Geometry: final body of the model. Coordinates: model frame, mm. A direction names the side the tool comes from. Coordinates: 2 decimals unless noted, no trailing zeros. Write each loop counter-clockwise with the first axis right and the second up, starting at its lowest first coordinate (ties: lowest second). Pieces come first, ordered by that corner, then holes.
from build123d import *

# Parameters (mm, degrees)
SKETCH_1_W          = 31
SKETCH_1_H          = 12.6
EXTRUDE_1_DEPTH     = 1
SKETCH_2_R          = 2.5
EXTRUDE_2_DEPTH     = 6
SKETCH_3_R          = 1.5
EXTRUDE_3_DEPTH     = 5.5
DOME_1_FACE_RADIUS  = 1.5
DOME_1_HEIGHT       = 0.5
DOME_2_FACE_RADIUS  = 1.5
DOME_2_HEIGHT       = 0.5
DOME_3_FACE_RADIUS  = 1.5
DOME_3_HEIGHT       = 0.5
SKETCH_4_R          = 1.5
CUT_EXTRUDE_1_DEPTH = 18.774701192
EXTRUDE_START       = 2
SKETCH_5_R          = 3
SKETCH_5_R_2        = 1.5
EXTRUDE_4_DEPTH     = 2
SKETCH_6_W          = 4.5
SKETCH_6_H          = 8
EXTRUDE_6_DEPTH     = 6
SKETCH_7_W          = 3.38323666
SKETCH_7_H          = 6.498483094
CUT_EXTRUDE_2_DEPTH = 5
FILLET_1_R          = 2
SKETCH_9_W          = 5.019385781
SKETCH_9_H          = 3.581166035
EXTRUDE_7_DEPTH     = 5


with BuildPart() as part:
    # 草图1 → 凸台-拉伸1 (new body)
    with BuildSketch(Plane(origin=(0, 0, 0), x_dir=(1, 0, 0), z_dir=(0, 1, 0))):
        Rectangle(SKETCH_1_W, SKETCH_1_H)
    extrude(amount=EXTRUDE_1_DEPTH)

    # 草图2 → 凸台-拉伸2 (add)
    with BuildSketch(Plane(origin=(0, 1, 0), x_dir=(1, 0, 0), z_dir=(0, 1, 0))):
        with Locations(Location((-10.5, 0, 0), (0, 0, 270))):
            Circle(SKETCH_2_R)
    extrude(amount=EXTRUDE_2_DEPTH)

    # 草图3 → 凸台-拉伸3 (add)
    with BuildSketch(Plane(origin=(0, 1, 0), x_dir=(1, 0, 0), z_dir=(0, 1, 0))):
        with Locations(Location((-13.5, -4.8, 0), (0, 0, 270))):
            Circle(SKETCH_3_R)
        with Locations(Location((-13.5, 4.8, 0), (0, 0, 90))):
            Circle(SKETCH_3_R)
        with Locations(Location((-5.186156124, 0, 0), (0, 0, 270))):
            Circle(SKETCH_3_R)
    extrude(amount=EXTRUDE_3_DEPTH)

    # 圆顶1: an elliptical dome of height H over a round flat face of radius A is half a spheroid: the quarter ellipse of half axes A and H revolved about the face's axis
    with BuildSketch(Plane((-13.5, 6.5, -4.8), x_dir=(0, 0, -1), z_dir=(1, 0, 0)), mode=Mode.PRIVATE) as dome_1_quarter:
        Ellipse(DOME_1_FACE_RADIUS, DOME_1_HEIGHT)
        Rectangle(DOME_1_FACE_RADIUS, DOME_1_HEIGHT, align=(Align.MIN, Align.MIN), mode=Mode.INTERSECT)
    revolve(dome_1_quarter.sketch, axis=Axis((-13.5, 6.5, -4.8), (0, 1, 0)))

    # 圆顶2: a dome of height H over a round flat face of radius A is a cap of a sphere of radius (A * A + H * H) / (2 * H)
    dome_2_r = (DOME_2_FACE_RADIUS * DOME_2_FACE_RADIUS + DOME_2_HEIGHT * DOME_2_HEIGHT) / (2 * DOME_2_HEIGHT)
    dome_2_base = Plane((-13.5, 6.5, 4.8), z_dir=(0, 1, 0))
    with Locations(dome_2_base.offset(DOME_2_HEIGHT - dome_2_r)):
        dome_2_ball = Sphere(dome_2_r, mode=Mode.PRIVATE)
    add(split(dome_2_ball, bisect_by=dome_2_base, keep=Keep.TOP, mode=Mode.PRIVATE))

    # 圆顶3: a dome of height H over a round flat face of radius A is a cap of a sphere of radius (A * A + H * H) / (2 * H)
    dome_3_r = (DOME_3_FACE_RADIUS * DOME_3_FACE_RADIUS + DOME_3_HEIGHT * DOME_3_HEIGHT) / (2 * DOME_3_HEIGHT)
    dome_3_base = Plane((-5.186156124, 6.5, 0), z_dir=(0, 1, 0))
    with Locations(dome_3_base.offset(DOME_3_HEIGHT - dome_3_r)):
        dome_3_ball = Sphere(dome_3_r, mode=Mode.PRIVATE)
    add(split(dome_3_ball, bisect_by=dome_3_base, keep=Keep.TOP, mode=Mode.PRIVATE))

    # 草图4 → 切除-拉伸1 (cut, through all)
    with BuildSketch(Plane(origin=(0, 1, 0), x_dir=(1, 0, 0), z_dir=(0, 1, 0))):
        with Locations(Location((6.5, 0, 0), (0, 0, 270))):
            Circle(SKETCH_4_R)
    extrude(amount=-CUT_EXTRUDE_1_DEPTH, mode=Mode.SUBTRACT)

    # 草图5 → 凸台-拉伸4 (add)
    with BuildSketch(Plane(origin=(0, 1, 0), x_dir=(1, 0, 0), z_dir=(0, 1, 0)).offset(EXTRUDE_START)):
        with Locations(Location((6.5, 0, 0), (0, 0, 270))):
            Circle(SKETCH_5_R)
        with Locations(Location((6.5, 0, 0), (0, 0, 270))):
            Circle(SKETCH_5_R_2, mode=Mode.SUBTRACT)
    extrude(amount=-EXTRUDE_4_DEPTH)

    # 草图6 → 凸台-拉伸6 (add)
    with BuildSketch(Plane(origin=(0, 0, 0), x_dir=(-1, 0, 0), z_dir=(0, -1, 0))):
        with Locations((-13.25, -0.193431005)):
            Rectangle(SKETCH_6_W, SKETCH_6_H)
    extrude(amount=EXTRUDE_6_DEPTH)

    # 草图7 → 切除-拉伸2 (cut)
    with BuildSketch(Plane.XZ.offset(6)):
        with Locations((13.25, 0.193431005)):
            Rectangle(SKETCH_7_W, SKETCH_7_H)
    extrude(amount=-CUT_EXTRUDE_2_DEPTH, mode=Mode.SUBTRACT)

    # 圆角1
    fillet_1_edges = [part.edges().sort_by_distance(p)[0] for p in [
        (-15.5, 0.5, -6.3),
        (-15.5, 0.5, 6.3),
    ]]
    fillet(fillet_1_edges, radius=FILLET_1_R)

    # 草图9 → 凸台-拉伸7 (add)
    with BuildSketch(Plane.XZ):
        with Locations((-1.930507992, 4.509416983)):
            Rectangle(SKETCH_9_W, SKETCH_9_H)
    extrude(amount=EXTRUDE_7_DEPTH)


solid = part.part
Item 1: Pull-direction query (Z, two-part tool) for faces 1 (the flat face through (13, -3, 4.193)), 2 (the flat face through (14.942, -4, 0)), 3 (the cylindrical face through (-14.93, 0.51, -5.7)), 4 (the cylindrical face through (-13.43, 3.71, 3.3)); classes: released by +Z, released by -Z, zero draft, split by the parting line, or undercut.
Derived:
face 1: released by +Z
face 2: undercut
face 3: released by -Z
face 4: undercut
Item 2: Material intervals for probe 1 along X at (y, z) = (1.45, 0); probe 2 along X at (y, z) = (-2.75, 4); probe 3 along X at (y, z) = (0.7, 0), sorted ascending.
Derived:
probe 1: x = -13 to -8, -6.69 to -3.69, 3.5 to 5, 8 to 9.5
probe 2: x = -4.44 to 0.58, 11 to 15.5
probe 3: x = -15.5 to 5, 8 to 15.5
Item 3: Pin query (flat end, axial travel): pin 1 (1.5 mm diameter, centred on x = 6, z = 1, fed in from +Y); pin 2 (4 mm diameter, centred on x = 6.5, z = 0, fed in from -Y); pin 3 (5.5 mm diameter, centred on y = -3, z = -1.5, fed in from -X). Return the tip coordinate at first contact, or that it passes through.
Derived:
pin 1: stops at y = 3
pin 2: stops at y = 0
pin 3: stops at x = 11
Item 4: Section A-A, the plane z = 0. Output: boundary loops of the cut face in (x, y).
Derived:
outline: (-15.5, 0) - (5, 0) - (5, 3) - (3.5, 3) - (3.5, 1) - (-3.69, 1) - (-3.69, 6.5) arc R2.5 ccw to (-6.69, 6.5) - (-6.69, 1) - (-8, 1) - (-8, 7) - (-13, 7) - (-13, 1) - (-15.5, 1) - close; (8, 0) - (11, 0) - (11, -6) - (11.56, -6) - (11.56, -1) - (14.94, -1) - (14.94, -6) - (15.5, -6) - (15.5, 1) - (9.5, 1) - (9.5, 3) - (8, 3) - close
Item 5: Section C-C, the plane y = -3.25. Output: boundary loops of the cut face in (x, z), plus the area to 3 significant figures.
Derived:
outline: (-4.44, 2.72) - (0.58, 2.72) - (0.58, 6.3) - (-4.44, 6.3) - close; (11, -3.81) - (15.5, -3.81) - (15.5, 4.19) - (11, 4.19) - close; hole (11.56, -3.06) - (14.94, -3.06) - (14.94, 3.44) - (11.56, 3.44) - close
area: 32.0 mm2
Item 6: Set-up query: faces 5 (the flat face through (13, -4, -3.056)), 6 (the cylindrical face through (-13.57, 3.71, -3.3)), 7 (the flat face through (0.579, -2, 4)). Return all of +Z, -Z, +X, -X, +Y, -Y with unobstructed straight access to the full face (end or side cutting, diameter ignored); none if empty.
Derived:
face 5: -Y
face 6: +Y
face 7: +Z, -Z, -Y
Item 7: Section B-B, the plane x = 6.5. Output: boundary loops of the cut face in (y, z).
Derived:
outline: (0, -6.3) - (1, -6.3) - (1, -3) - (3, -3) - (3, -1.5) - (0, -1.5) - close; (0, 1.5) - (3, 1.5) - (3, 3) - (1, 3) - (1, 6.3) - (0, 6.3) - close
Item 8: Section D-D, the plane x = -10.5. Output: boundary loops of the cut face in (y, z).
Derived:
outline: (0, -6.3) - (1, -6.3) - (1, -2.5) - (7, -2.5) - (7, 2.5) - (1, 2.5) - (1, 6.3) - (0, 6.3) - close
